from build123d import *

# Parameters (mm, degrees)
SKETCH_1_R          = 4
EXTRUDE_1_DEPTH     = 30
CUT_EXTRUDE_1_DEPTH = 20
FILLET_1_R          = 8
SKETCH_3_R          = 4
CUT_EXTRUDE_2_DEPTH = 41


with BuildPart() as part:
    # 스케치1 → 보스-돌출1 (new body)
    with BuildSketch(Plane(origin=(0, 0, 0), x_dir=(1, 0, 0), z_dir=(0, 1, 0))):
        with BuildLine():
            Line((-30, -20), (30, -20))
            ThreePointArc((30, -20), (37.071067812, -17.071067812), (40, -10))
            Line((40, -10), (40, 20))
            Line((40, 20), (-40, 20))
            Line((-40, 20), (-40, -10))
            ThreePointArc((-40, -10), (-37.071067812, -17.071067812), (-30, -20))
        make_face()
        with Locations(Location((-30, -10, 0), (0, 0, 270))):  # turned: the seam where the file's is
            Circle(SKETCH_1_R, mode=Mode.SUBTRACT)
        with Locations(Location((30, -10, 0), (0, 0, 270))):  # turned: the seam where the file's is
            Circle(SKETCH_1_R, mode=Mode.SUBTRACT)
    extrude(amount=EXTRUDE_1_DEPTH)

    # 스케치2 → 컷-돌출1 (cut)
    with BuildSketch(Plane(origin=(0, 30, 0), x_dir=(1, 0, 0), z_dir=(0, 1, 0))):
        with BuildLine():
            Line((40, -10), (40, 10))
            Line((40, 10), (20, 10))
            Line((20, 10), (20, -15))
            Line((20, -15), (-20, -15))
            Line((-20, -15), (-20, 10))
            Line((-20, 10), (-40, 10))
            Line((-40, 10), (-40, -10))
            ThreePointArc((-40, -10), (-37.071067812, -17.071067812), (-30, -20))
            Line((-30, -20), (30, -20))
            ThreePointArc((30, -20), (37.071067812, -17.071067812), (40, -10))
        make_face()
    extrude(amount=-CUT_EXTRUDE_1_DEPTH, mode=Mode.SUBTRACT)

    # 필렛1
    fillet_1_edges = [part.edges().sort_by_distance(p)[0] for p in [
        (-40, 30, -15),
        (40, 30, -15),
    ]]
    fillet(fillet_1_edges, radius=FILLET_1_R)

    # 스케치3 → 컷-돌출2 (cut, through all)
    with BuildSketch(Plane.XY.offset(20)):
        with Locations((-32, 22)):
            Circle(SKETCH_3_R)
        with Locations((32, 22)):
            Circle(SKETCH_3_R)
        with BuildLine():
            Line((15, 30), (-15, 30))
            ThreePointArc((-15, 30), (0, 15), (15, 30))
        make_face()
    extrude(amount=-CUT_EXTRUDE_2_DEPTH, mode=Mode.SUBTRACT)


solid = part.part
Design review of the part built by this model. Coordinates are the model's own, in mm. A direction names the side the tool comes from. Round coordinates to 2 decimals unless told otherwise and drop trailing zeros. Write each loop counter-clockwise with the first axis right and the second up, starting at its lowest first coordinate (ties: lowest second). Pieces come first, ordered by that corner, then holes. Notation, with made-up numbers: (10, -3.5) -> (54, -3.5) arc R13 ccw to (54, 16.5) -> close; hole circle Ø9 at (2.5, 18.5). An arc over 180 degrees is marked (long way). One line per question, with ' | ' between items.
(1) Machinability: for faces 1 (the flat face through (30, 18, -10)), 2 (the flat face through (0, 5, 20)), 3 (the flat face through (0, 13, 15)), 4 (the flat face through (-28, 20, -10)), which of the approach directions +Z, -Z, +X, -X, +Y, -Y give a long, thin tool a straight path to every point of the face, cutting with its end or side? Answer none if there is none.
Result sheet:
face 1: +Z, +X, +Y | face 2: +Z, +X, -X, +Y, -Y | face 3: +Z, +X, -X, +Y | face 4: +Z, -X, +Y
(2) Take a section at C-C, the plane x = 0. State the section outline as (y, z) points, and give its area (3 significant figures).
Result sheet:
outline: (0, -20) -> (15, -20) -> (15, 15) -> (10, 15) -> (10, 20) -> (0, 20) -> close | area: 575 mm2
(3) Insertion check: P1, Ø10, axis at x = -3, z = -14, coming from the -Y side; P2, Ø9, axis at x = 30, z = 10, coming from the +Y side; P3, Ø10, axis at y = 22, z = 5.5, coming from the +X side; P4, Ø6.5, axis at x = -32, y = 22, coming from the -Z side. Each pin has a flat end and moves straight along its axis. Give the tip position at first contact, or say it passes through.
Result sheet:
P1: y = 0 | P2: y = 10 | P3: x = 20 | P4: through
(4) Take a section at A-A, the plane y = 23.5. State the section outline as (x, z) points, and give its area (3 significant figures).
Result sheet:
outline: (-39.86, -20) -> (-35.71, -20) -> (-35.71, -10) -> (-39.86, -10) -> close; (-28.29, -20) -> (-13.52, -20) -> (-13.52, 15) -> (-20, 15) -> (-20, -10) -> (-28.29, -10) -> close; (13.52, -20) -> (28.29, -20) -> (28.29, -10) -> (20, -10) -> (20, 15) -> (13.52, 15) -> close; (35.71, -20) -> (39.86, -20) -> (39.86, -10) -> (35.71, -10) -> close | area: 703 mm2
(5) Take a section at D-D, the plane z = -3. State the section outline as (x, y) points, and give its area (3 significant figures).
Result sheet:
outline: (-40, 0) -> (40, 0) -> (40, 10) -> (20, 10) -> (20, 30) -> (15, 30) arc R15 cw to (-15, 30) -> (-20, 30) -> (-20, 10) -> (-40, 10) -> close | area: 1,250 mm2
(6) Take a section at B-B, the plane y = 4.5. State the section outline as (x, z) points.
Result sheet:
outline: (-40, -20) -> (40, -20) -> (40, 10) arc R10 ccw to (30, 20) -> (-30, 20) arc R10 ccw to (-40, 10) -> close; hole circle Ø8 at (-30, 10); hole circle Ø8 at (30, 10)
(7) Draft analysis for pull direction Z (two halves, no side actions). For faces 5 (the cylindrical face through (36.99, 4.93, 17.15)), 6 (the flat face through (20, 20, 2)), 7 (the cylindrical face through (-26.034, 4.93, 9.479)), state which applies: released by +Z, released by -Z, zero draft, split by the parting line, or undercut.
Result sheet:
face 5: released by +Z | face 6: zero draft | face 7: undercut
(8) Wall thickness on line 1 (X direction, y = 7, z = 10); line 2 (Z direction, x = 30, y = 5.5); line 3 (X direction, y = 18.5, z = -15): over which ranges is each line inside the solid? List them lowest first. Write a range as [from, to].
Result sheet:
line 1: [-40, -34], [-26, 26], [34, 40] | line 2: [-20, 6], [14, 20] | line 3: [-40, -33.94], [-30.06, -9.63], [9.63, 30.06], [33.94, 40]
